For this review, take the finished solid that the model builds, in its own axes (mm). Face numbers are marked on the shaded views. A direction names the side the tool comes from. Give positions to 0.01 mm unless a question says otherwise; leave off trailing zeros. Write each loop counter-clockwise with the first axis right and the second up, starting at its lowest first coordinate (ties: lowest second). Pieces come first, ordered by that corner, then holes. Notation, with made-up numbers: M 28,54 L 56,54 A19 ccw 56,88 Z; hole C 56.5,70.25 d9. An arc over 180 degrees is marked long. Answer as a JSON object with one key per item and string values. Group by question number.
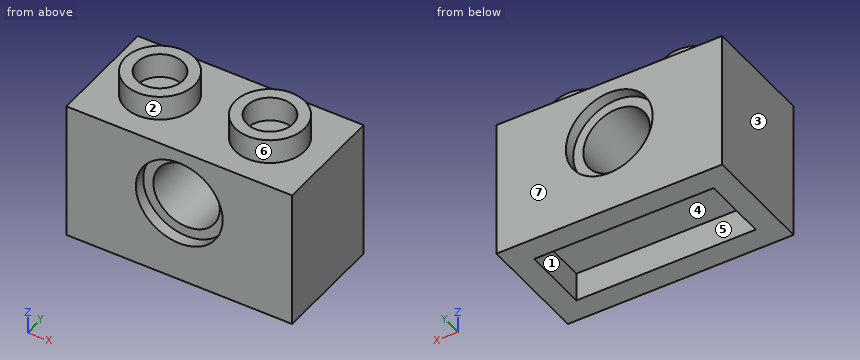
```python
from build123d import *

# Parameters (mm, degrees)
F0_W     = 15.6
F0_H     = 9.6
F0_R     = 3
F0_R_2   = 2.3
F1_DEPTH = 7.8
F2_R     = 2.4
F2_R_2   = 1.6
F3_DEPTH = 1.7
F5_DEPTH = 2
F6_DEPTH = 0.8
F7_R     = 3
F7_R_2   = 2.3
F8_DEPTH = 0.8


with BuildPart() as f1:
    # F0 (on Front) → F1 (new body)
    with BuildSketch(Plane.XZ):
        with Locations((-5.3637987003, 2.2607615549)):
            Rectangle(F0_W, F0_H)
        with Locations((-5.3637987003, 3.1607615549)):
            Circle(F0_R, mode=Mode.SUBTRACT)
        with Locations((-5.3637987003, 3.1607615549)):
            Circle(F0_R)
        with Locations((-5.3637987003, 3.1607615549)):
            Circle(F0_R_2, mode=Mode.SUBTRACT)
    extrude(amount=F1_DEPTH)

    # F2 (on face) → F3 (join)
    with BuildSketch(Plane.XY.offset(7.0607615549)):
        with Locations((-1.5637987003, -3.9)):
            Circle(F2_R)
        with Locations((-1.5637987003, -3.9)):
            Circle(F2_R_2, mode=Mode.SUBTRACT)
        with Locations((-9.1637987003, -3.9)):
            Circle(F2_R)
        with Locations((-9.1637987003, -3.9)):
            Circle(F2_R_2, mode=Mode.SUBTRACT)
    extrude(amount=F3_DEPTH)

    # F4 (on face) → F5 (cut)
    with BuildSketch(Plane(origin=(0, 0, -2.5392384451), x_dir=(1, 0, 0), z_dir=(0, 0, -1))):
        Polygon((-11.5637987003, 6.2), (-11.5637987003, 3.9), (-11.5637987003, 1.6), (-5.3637987003, 1.6), (0.8362012997, 1.6), (0.8362012997, 3.9), (0.8362012997, 6.2), (-5.3637987003, 6.2), align=None)
    extrude(amount=-F5_DEPTH, mode=Mode.SUBTRACT)

    # F0 (on Front) → F6 (cut)
    with BuildSketch(Plane.XZ):
        with Locations((-5.3637987003, 3.1607615549)):
            Circle(F0_R)
        with Locations((-5.3637987003, 3.1607615549)):
            Circle(F0_R_2, mode=Mode.SUBTRACT)
    extrude(amount=F6_DEPTH, mode=Mode.SUBTRACT)

    # F7 (on face) → F8 (cut)
    with BuildSketch(Plane.XZ.offset(7.8)):
        with Locations((-5.3637987003, 3.1607615549)):
            Circle(F7_R)
        with Locations((-5.3637987003, 3.1607615549)):
            Circle(F7_R_2, mode=Mode.SUBTRACT)
    extrude(amount=-F8_DEPTH, mode=Mode.SUBTRACT)


solid = f1.part
```
Item 1: Consider section D-D (z = 7.5). Give the boundary of the cut face in (x, y), plus the area to 3 significant figures.
Item 2: Consider section B-B (x = -5.25). Give the boundary of the cut face in (y, z), plus the area to 3 significant figures.
Item 3: Consider section C-C (y = -3.25). Give the boundary of the cut face in (x, z).
Item 4: To check wall thickness, follow probe 1 along X at (y, z) = (-6, -0.75); probe 2 along Y at (x, z) = (-6.25, -1.75); probe 3 along Z at (x, y) = (-11.5, -6). State the ranges of each line that lie inside material, in increasing order.
Item 5: Consider section A-A (z = 4). Give the boundary of the cut face in (x, y).
Item 6: Draft analysis for pull direction Y (two halves, no side actions). For the marked faces 1, 2, 3 and 4, state which applies: released by +Y, released by -Y, zero draft, split by the parting line, or undercut.
Item 7: Insertion check: P1, Ø2.5, axis at x = -4, y = -5, coming from the -Z side; P2, Ø5.5, axis at x = -5.36, z = 3.16, coming from the -Y side; P3, Ø3, axis at x = -6, z = 4, coming from the +Y side; P4, Ø1.6, axis at x = -9, y = -4.5, coming from the +Z side. Each pin has a flat end and moves straight along its axis. Give the tip position at first contact, or say it passes through.
Item 8: Machinability: for the marked faces 5, 6 and 7, which of the approach directions +Z, -Z, +X, -X, +Y, -Y give a long, thin tool a straight path to every point of the face, cutting with its end or side? Answer none if there is none.
Result set:
{
 "1": {"outline": "C -9.16,-3.9 d4.8; C -1.56,-3.9 d4.8; hole C -9.16,-3.9 d3.2; hole C -1.56,-3.9 d3.2", "area": "20.1 mm^2"},
 "2": {"outline": "M -7.8,-2.54 L -6.2,-2.54 L -6.2,-0.54 L -1.6,-0.54 L -1.6,-2.54 L 0,-2.54 L 0,0.16 L -0.8,0.16 L -0.8,0.86 L -7,0.86 L -7,0.16 L -7.8,0.16 Z; M -7.8,6.16 L -7,6.16 L -7,5.46 L -0.8,5.46 L -0.8,6.16 L 0,6.16 L 0,7.06 L -7.8,7.06 Z", "area": "27.6 mm^2"},
 "3": {"outline": "M -13.16,-2.54 L -11.56,-2.54 L -11.56,-0.54 L 0.84,-0.54 L 0.84,-2.54 L 2.44,-2.54 L 2.44,7.06 L 0.75,7.06 L 0.75,8.76 L -0.1,8.76 L -0.1,7.06 L -3.03,7.06 L -3.03,8.76 L -3.87,8.76 L -3.87,7.06 L -6.85,7.06 L -6.85,8.76 L -7.7,8.76 L -7.7,7.06 L -10.63,7.06 L -10.63,8.76 L -11.47,8.76 L -11.47,7.06 L -13.16,7.06 Z; hole C -5.36,3.16 d4.6"},
 "4": {"probe 1": "x = -13.16 to -11.56, 0.84 to 2.44", "probe 2": "y = -7.8 to -6.2, -1.6 to 0", "probe 3": "z = -0.54 to 7.06"},
 "5": {"outline": "M -13.16,-7.8 L -8.24,-7.8 L -8.24,-7 L -7.51,-7 L -7.51,-0.8 L -8.24,-0.8 L -8.24,0 L -13.16,0 Z; M -3.22,-7 L -2.48,-7 L -2.48,-7.8 L 2.44,-7.8 L 2.44,0 L -2.48,0 L -2.48,-0.8 L -3.22,-0.8 Z"},
 "6": {"face 1": "undercut", "face 2": "split by the parting line", "face 3": "zero draft", "face 4": "undercut"},
 "7": {"P1": "stops at z = -2.54", "P2": "stops at y = -7", "P3": "stops at y = -0.8", "P4": "stops at z = 7.06"},
 "8": {"face 5": "-Z", "face 6": "+Z", "face 7": "+Z, -Z, +X, -X, +Y"}
}
